Check sheet for the drawn part. Datum: minimum x, y, z corner. Units: mm. A direction names the side the tool comes from. Give positions to 0.01 mm unless a question says otherwise; leave off trailing zeros. Order: outer loops, then holes, each group sorted by start corner. A loop starts at its lowest first (then second) coordinate and runs counter-clockwise, first axis right, second up. Notation, with made-up numbers: M 58,-2.5 L 93,-2.5 A11 cw 93,3.5 Z; hole C 38,24 d9. An arc over 180 degrees is marked long. One line per question, with ' | ' between items. Start each with the question number.
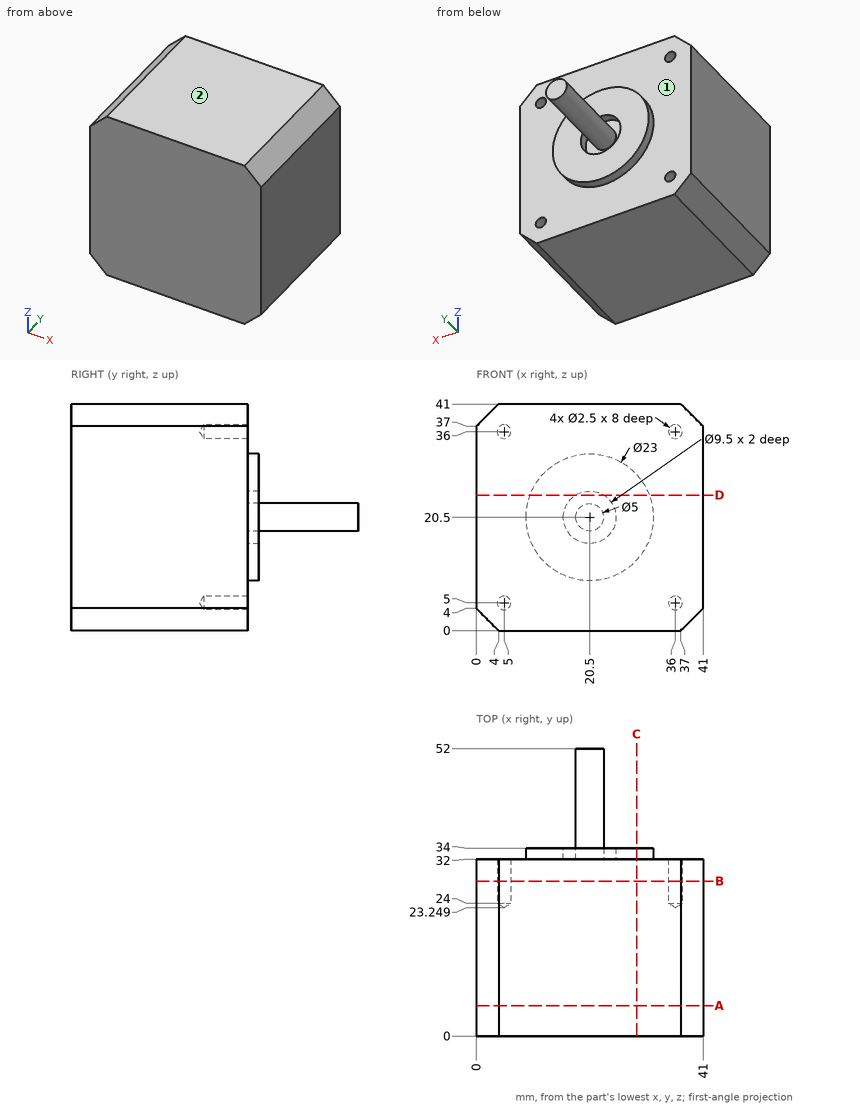
Item 1: Section check D-D, the plane z = 24.5. Record the cut outline in (x, y).
Item 2: Section check A-A, the plane y = 5.5. Record the cut outline in (x, z).
Item 3: Set-up check for the marked faces 1 and 2: record each of +Z, -Z, +X, -X, +Y, -Y from which the full face is reachable in a straight line by a thin tool's end or side.
Item 4: Scan line: probe 1 along Z at (x, y) = (36, 28). Record every from-to range of solid material in increasing order. Write a range as [from, to].
Item 5: Section check C-C, the plane x = 29. Record the cut outline in (y, z), then the cut area to 3 significant figures.
Item 6: Section check B-B, the plane y = 28. Record the cut outline in (x, z).
Item 7: Go/stop test with flat-tipped pins: P1, Ø18.5, axis at x = 20.5, z = 23.5, coming from the +Y side; P2, Ø12, axis at x = 32.5, z = 31.5, coming from the +Y side; P3, Ø4, axis at x = 36, z = 36, coming from the +Y side; P4, Ø1.5, axis at x = 5, z = 5, coming from the +Y side. Record where each tip stops, or that it passes through.
Reported:
1) outline: M 0,0 L 41,0 L 41,32 L 31.28,32 L 31.28,34 L 23.06,34 L 23.06,32 L 17.94,32 L 17.94,34 L 9.72,34 L 9.72,32 L 0,32 Z
2) outline: M 0,4 L 4,0 L 37,0 L 41,4 L 41,37 L 37,41 L 4,41 L 0,37 Z
3) face 1: +Y | face 2: +Z, +X, -X, +Y, -Y
4) probe 1: z = [0, 3.75], [6.25, 34.75], [37.25, 41]
5) outline: M 0,0 L 32,0 L 32,12.75 L 34,12.75 L 34,28.25 L 32,28.25 L 32,41 L 0,41 Z | area: 1,340 mm^2
6) outline: M 0,4 L 4,0 L 37,0 L 41,4 L 41,37 L 37,41 L 4,41 L 0,37 Z; hole C 5,5 d2.5; hole C 5,36 d2.5; hole C 36,5 d2.5; hole C 36,36 d2.5
7) P1: stops at y = 52 | P2: stops at y = 34 | P3: stops at y = 32 | P4: stops at y = 23.7
